from build123d import *

# Parameters (mm, degrees)
AUFSATZ_LINEAR_AUSTRAGEN1_DEPTH      = 10.85
AUFSATZ_LINEAR_AUSTRAGEN1_DEPTH_BACK = 10.85
SKIZZE3_W                            = 46.7
SKIZZE3_H                            = 6
SCHNITT_LINEAR_START                 = 618
SKIZZE4_R                            = 4.5
SKIZZE4_R_2                          = 1.5
SCHNITT_LINEAR_AUSTRAGEN1_DEPTH      = 10
SCHNITT_LINEAR_START_2               = 10.85
SKIZZE6_R                            = 1.25
SCHNITT_LINEAR_AUSTRAGEN2_DEPTH      = 6
SCHNITT_LINEAR_START_3               = -4.85
SKIZZE6_2_R                          = 1.25
SCHNITT_LINEAR_AUSTRAGEN3_DEPTH      = 6
SCHNITT_LINEAR_START_4               = 612
SCHNITT_LINEAR_AUSTRAGEN4_DEPTH      = 6


# Read off the part's stored shape, not the designer's step: Schnitt-Linear austragen4
with BuildPart() as part:
    # Skizze3 → Aufsatz-Linear austragen1 (new, two sides: drawn at the far end of the back side and taken through both)
    with BuildSketch(Plane.XY.offset(-AUFSATZ_LINEAR_AUSTRAGEN1_DEPTH_BACK)):
        with Locations((0, 615)):
            Rectangle(SKIZZE3_W, SKIZZE3_H)
    extrude(amount=AUFSATZ_LINEAR_AUSTRAGEN1_DEPTH + AUFSATZ_LINEAR_AUSTRAGEN1_DEPTH_BACK)

    # Skizze4 → Schnitt-Linear austragen1 (cut)
    with BuildSketch(Plane(origin=(0, 0, 0), x_dir=(1, 0, 0), z_dir=(0, 1, 0)).offset(SCHNITT_LINEAR_START)):
        with Locations(Location((0, 0, 0), (0, 0, 270))):
            Circle(SKIZZE4_R)
        with Locations(Location((14, 0, 0), (0, 0, 270))):
            Circle(SKIZZE4_R_2)
    extrude(amount=-SCHNITT_LINEAR_AUSTRAGEN1_DEPTH, mode=Mode.SUBTRACT)

    # Skizze6 → Schnitt-Linear austragen2 (cut)
    with BuildSketch(Plane.XY.offset(SCHNITT_LINEAR_START_2)):
        with Locations(Location((18.35, 615, 0), (0, 0, 180))):
            Circle(SKIZZE6_R)
        with Locations(Location((-8, 615, 0), (0, 0, 180))):
            Circle(SKIZZE6_R)
    extrude(amount=-SCHNITT_LINEAR_AUSTRAGEN2_DEPTH, mode=Mode.SUBTRACT)

    # Skizze6<2> → Schnitt-Linear austragen3 (cut)
    with BuildSketch(Plane.XY.offset(SCHNITT_LINEAR_START_3)):
        with Locations((18.35, 234)):
            Circle(SKIZZE6_2_R)
        with Locations((-8, 234)):
            Circle(SKIZZE6_2_R)
        with Locations(Location((18.35, 615, 0), (0, 0, 180))):
            Circle(SKIZZE6_2_R)
        with Locations(Location((-8, 615, 0), (0, 0, 180))):
            Circle(SKIZZE6_2_R)
    extrude(amount=-SCHNITT_LINEAR_AUSTRAGEN3_DEPTH, mode=Mode.SUBTRACT)

    # Schnitt-Linear austragen4 outline → Schnitt-Linear austragen4 (cut)
    with BuildSketch(Plane(origin=(0, 0, 0), x_dir=(1, 0, 0), z_dir=(0, 1, 0)).offset(SCHNITT_LINEAR_START_4)):
        with BuildLine():
            Line((-23.35, 10.85), (-23.35, 1.469693846))
            ThreePointArc((-23.35, 1.469693846), (-19.733593827, 8.17522716), (-12.6, 10.85))
            Line((-12.6, 10.85), (-23.35, 10.85))
        make_face()
        with BuildLine():
            ThreePointArc((-12.6, -10.85), (-19.733593827, -8.17522716), (-23.35, -1.469693846))
            Line((-23.35, -1.469693846), (-23.35, -10.85))
            Line((-23.35, -10.85), (-12.6, -10.85))
        make_face()
    extrude(amount=SCHNITT_LINEAR_AUSTRAGEN4_DEPTH, mode=Mode.SUBTRACT)


solid = part.part
For this review, take the finished solid that the model builds, in its own axes (mm). A direction names the side the tool comes from. Round coordinates to 2 decimals unless told otherwise and drop trailing zeros. Write each loop counter-clockwise with the first axis right and the second up, starting at its lowest first coordinate (ties: lowest second). Pieces come first, ordered by that corner, then holes. Notation, with made-up numbers: (28, 62.5) - (43, 62.5) arc R27 ccw to (43, 99.5) - close; hole circle Ø6 at (14, 0). An arc over 180 degrees is marked (long way). Write item = value, one per line. Start each with the question number.
1. Consider section D-D on x = -8. State the section outline as (y, z) points.
2. Consider section C-C on y = 615. State the section outline as (x, z) points, plus the area to 3 significant figures.
3. Consider section A-A on x = 0. State the section outline as (y, z) points, plus the area to 3 significant figures.
4. For faces 1 (the face through (5, 612, 0)), 2 (the face through (18, 615, -4.85)), 3 (the face through (-8, 615, 4.85)), list the 3-axis set-ups (+Z, -Z, +X, -X, +Y, -Y) from which the entire face can be reached by the end or side of a thin tool; tool diameter is ignored.
5. Wall thickness on L1, parallel to X at y = 616.4, z = 0; L2, parallel to X at y = 615, z = 9.6; L3, parallel to Y at x = 18.35, z = -8.55: over which ranges is each line inside the solid? List them lowest first.
6. Consider section B-B on z = 0. State the section outline as (x, y) points.
7. For pin 1 Ø2 at (x, y) = (-8, 615) entering from +Z; pin 2 Ø1.5 at (y, z) = (615, 4.5) entering from -X; pin 3 Ø3 at (x, y) = (18.5, 614.5) entering from -Z, all flat-tipped, find the tip position at first contact; note any pin that passes through.
8. Draft analysis for pull direction Y (two halves, no side actions). For faces 4 (the face through (5, 618, 0)), 5 (the face through (1.352, 615.042, 4.292)), 6 (the face through (-7.84, 613.76, 7.89)), state which applies: released by +Y, released by -Y, zero draft, split by the parting line, or undercut.
Evaluation:
q1.outline = (612, -10.85) - (613.75, -10.85) - (613.75, -4.85) - (616.25, -4.85) - (616.25, -10.85) - (618, -10.85) - (618, 10.85) - (616.25, 10.85) - (616.25, 4.85) - (613.75, 4.85) - (613.75, 10.85) - (612, 10.85) - close
q2.outline = (-23.35, -1.47) arc R10.85 ccw to (-12.6, -10.85) - (-9.25, -10.85) - (-9.25, -4.85) - (-6.75, -4.85) - (-6.75, -10.85) - (17.1, -10.85) - (17.1, -4.85) - (19.6, -4.85) - (19.6, -10.85) - (23.35, -10.85) - (23.35, 10.85) - (19.6, 10.85) - (19.6, 4.85) - (17.1, 4.85) - (17.1, 10.85) - (-6.75, 10.85) - (-6.75, 4.85) - (-9.25, 4.85) - (-9.25, 10.85) - (-12.6, 10.85) arc R10.85 ccw to (-23.35, 1.47) - close; hole circle Ø9 at (0, 0); hole circle Ø3 at (14, 0)
q2.area = 834 mm2
q3.outline = (612, -10.85) - (618, -10.85) - (618, -4.5) - (612, -4.5) - close; (612, 4.5) - (618, 4.5) - (618, 10.85) - (612, 10.85) - close
q3.area = 76.2 mm2
q4.face_1 = +Z, -Z, +X, -X, -Y
q4.face_2 = -Z
q4.face_3 = +Z
q5.L1 = -23.35 to -4.5, 4.5 to 12.5, 15.5 to 23.35
q5.L2 = -17.66 to -9.25, -6.75 to 17.1, 19.6 to 23.35
q5.L3 = 612 to 613.75, 616.25 to 618
q6.outline = (-23.35, 612) - (-4.5, 612) - (-4.5, 618) - (-23.35, 618) - close; (4.5, 612) - (12.5, 612) - (12.5, 618) - (4.5, 618) - close; (15.5, 612) - (23.35, 612) - (23.35, 618) - (15.5, 618) - close
q7.pin_1 = 4.85
q7.pin_2 = -22.78
q7.pin_3 = -10.85
q8.face_4 = released by +Y
q8.face_5 = zero draft
q8.face_6 = undercut
